Could you check a few things on this drawing? It's one solid part, dimensions in mm from its lowest x, y, z. A direction names the side the tool comes from. Give positions to 0.01 mm unless a question says otherwise; leave off trailing zeros. Order: outer loops, then holes, each group sorted by start corner. A loop starts at its lowest first (then second) coordinate and runs counter-clockwise, first axis right, second up.
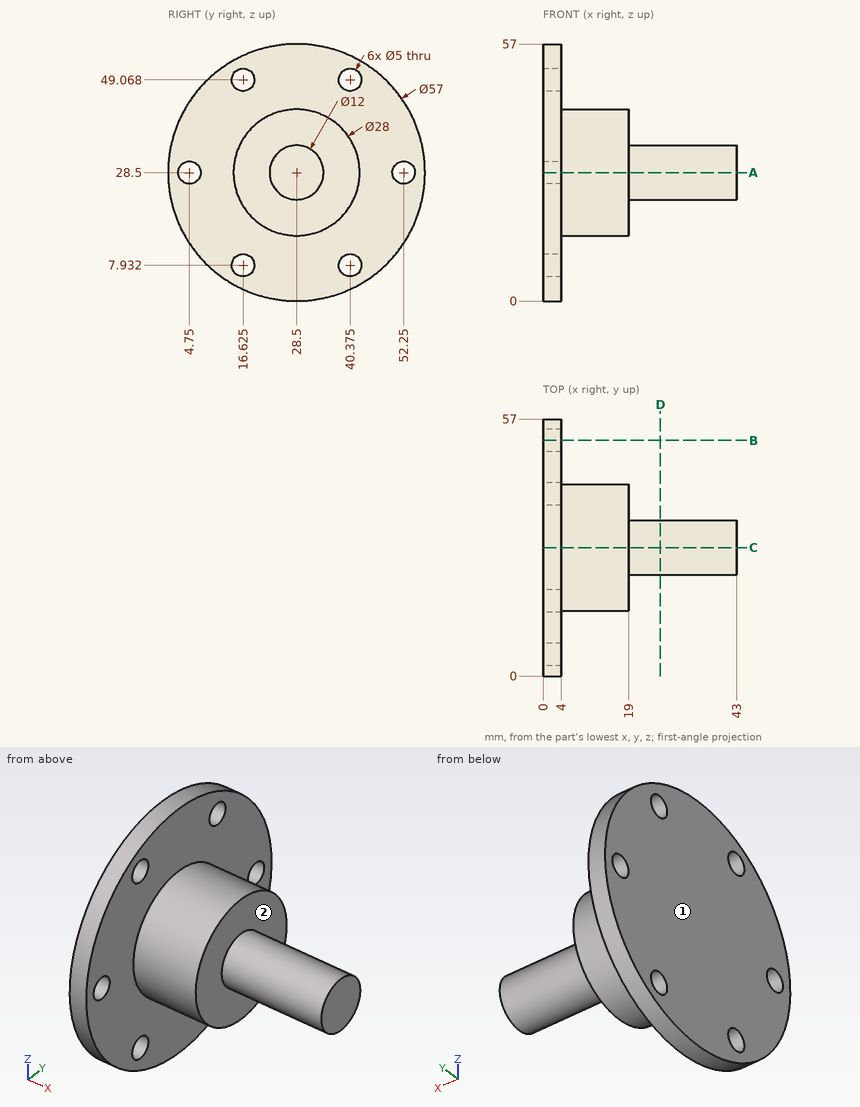
Q1. If we section it at A-A on z = 28.5: List the corners of the cut face in (x, y) for me, plus the area to 3 significant figures.
Filled sheet:
outline: (0, 0) - (4, 0) - (4, 2.25) - (0, 2.25) - close; (0, 7.25) - (4, 7.25) - (4, 14.5) - (19, 14.5) - (19, 22.5) - (43, 22.5) - (43, 34.5) - (19, 34.5) - (19, 42.5) - (4, 42.5) - (4, 49.75) - (0, 49.75) - close; (0, 54.75) - (4, 54.75) - (4, 57) - (0, 57) - close
area: 896 mm2
Q2. If we section it at D-D on x = 26: List the corners of the cut face in (y, z) for me.
Filled sheet:
outline: circle Ø12 at (28.5, 28.5)
Q3. For the marked faces 1 and 2, which set-ups out of +Z, -Z, +X, -X, +Y, -Y let a thin tool reach every point of the face, with its end or its side?
Filled sheet:
face 1: +Z, -Z, -X, +Y, -Y
face 2: +X
Q4. If we section it at B-B on y = 52.25: List the corners of the cut face in (x, z) for me, plus the area to 3 significant figures.
Filled sheet:
outline: (0, 12.75) - (4, 12.75) - (4, 26) - (0, 26) - close; (0, 31) - (4, 31) - (4, 44.25) - (0, 44.25) - close
area: 106 mm2
Q5. If we section it at C-C on y = 28.5: List the corners of the cut face in (x, z) for me.
Filled sheet:
outline: (0, 0) - (4, 0) - (4, 14.5) - (19, 14.5) - (19, 22.5) - (43, 22.5) - (43, 34.5) - (19, 34.5) - (19, 42.5) - (4, 42.5) - (4, 57) - (0, 57) - close
Q6. I need wall thicknesses on L1, parallel to Y at x = 2.65, z = 28.5; L2, parallel to Y at x = 2, z = 8; L3, parallel to X at y = 7, z = 10. Which ranges of each line are inside material? Lowest first, please.
Filled sheet:
L1: y = 0 to 2.25, 7.25 to 49.75, 54.75 to 57
L2: y = 8.7 to 14.13, 19.12 to 37.88, 42.87 to 48.3
L3: x = 0 to 4
Q7. I'm going to push flat-ended pins straight in: P1, Ø8, axis at x = 12, z = 18, coming from the +Y side; P2, Ø12, axis at x = 33.5, y = 26.5, coming from the -Z side; P3, Ø8, axis at y = 47, z = 14, coming from the +X side; P4, Ø6, axis at y = 40.38, z = 7.93, coming from the -X side. Where does each tip first touch, or does it pass through?
Filled sheet:
P1: stops at y = 40.9
P2: stops at z = 22.5
P3: stops at x = 4
P4: stops at x = 0
